Part model, mm, in its own coordinate system. Coordinates: 2 decimals unless noted, no trailing zeros. Write each loop counter-clockwise with the first axis right and the second up, starting at its lowest first coordinate (ties: lowest second). Pieces come first, ordered by that corner, then holes. Notation, with made-up numbers: (79.5, 69.25) - (86.5, 69.25) arc R26 ccw to (86.5, 83.25) - close; hole circle Ø8 at (39.5, -7.5). An arc over 180 degrees is marked (long way). Use a Markdown table: item, result.
Autodesk Inventor part; units mm, degrees
ref_plane "YZ Plane" through (0, 0, 0) normal (1, 0, 0) x (0, 1, 0)
ref_plane "XZ Plane" through (0, 0, 0) normal (0, 1, 0) x (-1, 0, 0)
ref_plane "XY Plane" through (0, 0, 0) normal (0, 0, 1) x (1, 0, 0)
sketch "Sketch1" plane through (0, 0, 0) normal (0, 1, 0) x (-1, 0, 0)
  circle A0 centre (0, 0) radius 8
  dimension "d0" = 16
extrude "Extrusion1" add sketch "Sketch1" along normal blind 31.5
sketch "Sketch2" plane through (0, 31.5, 0) normal (0, 1, 0) x (1, 0, 0)
  circle A0 centre (0, 0) radius 8
  circle A1 centre (0, 3.75) radius 0.4
  circle A2 centre (0, -3.75) radius 0.4
  dimension "d3" = 0.8
  dimension "d4" = 0.8
  dimension "d5" = 3.75
  dimension "d6" = 3.75
extrude "Extrusion2" add sketch "Sketch2" along normal blind 15 contours A1 | A2
fillet "Fillet1" radius 2 1 edges at (8, 0, 0)
fillet "Fillet2" radius 1 1 edges at (8, 31.5, 0)
properties part number "Capacitor"
Item 1: Drop flat-ended pins along their axis: P1, Ø5, axis at x = -3, z = 4.5, coming from the +Y side; P2, Ø1.5, axis at x = -1.5, y = 6.5, coming from the -Z side; P3, Ø4, axis at y = 7, z = 3.5, coming from the -X side. Give the stop position or say it passes through.
From the geometry:
| item | result |
|---|---|
| P1 | y = 31.5 |
| P2 | z = -7.96 |
| P3 | x = -7.86 |
Item 2: Band-saw the part on D-D, the plane y = 31. Give the cut face in (x, z), then the cut area to 3 significant figures.
From the geometry:
| item | result |
|---|---|
| outline | circle Ø15.73 at (0, 0) |
| area | 194 mm^2 |
Item 3: Two-plate mould, pull along Z, no slides. Class faces 1 (the face through (0, 0, 0)), 2 (the face through (1.73, 16.05, 7.81)), 3 (the face through (-0.052, 38.895, 4.147)): pulls with the +Z half, pulls with the -Z half, needs draft (parallel to the pull), parting line crosses it, or undercut.
From the geometry:
| item | result |
|---|---|
| face 1 | needs draft |
| face 2 | parting line crosses it |
| face 3 | undercut |
Item 4: Drill centre lines: probe 1 along Y at (x, z) = (2.5, 4); probe 2 along X at (y, z) = (3, 0.75); probe 3 along X at (y, z) = (36.5, 3.5). Where is each one in solid material? Low to high.
From the geometry:
| item | result |
|---|---|
| probe 1 | 0 to 31.5 |
| probe 2 | -7.96 to 7.96 |
| probe 3 | -0.31 to 0.31 |
Item 5: Band-saw the part on B-B, the plane y = 41. Give the cut face in (x, z), then the cut area to 3 significant figures.
From the geometry:
| item | result |
|---|---|
| outline | circle Ø0.8 at (0, -3.75); circle Ø0.8 at (0, 3.75) |
| area | 1.01 mm^2 |
Item 6: Band-saw the part on C-C, the plane y = 15. Give the cut face in (x, z).
From the geometry:
| item | result |
|---|---|
| outline | circle Ø16 at (0, 0) |
Item 7: Band-saw the part on A-A, the plane z = 0. Give the cut face in (x, y), then the cut area to 3 significant figures.
From the geometry:
| item | result |
|---|---|
| outline | (-8, 2) arc R2 ccw to (-6, 0) - (6, 0) arc R2 ccw to (8, 2) - (8, 30.5) arc R1 ccw to (7, 31.5) - (-7, 31.5) arc R1 ccw to (-8, 30.5) - close |
| area | 502 mm^2 |
